The listing builds one solid part. Answer for the finished solid, in the listing's coordinates (mm). Face numbers are marked on the shaded views. A direction names the side the tool comes from. Round coordinates to 2 decimals unless told otherwise and drop trailing zeros. Order: outer loops, then holes, each group sorted by start corner. A loop starts at its lowest first (then second) coordinate and runs counter-clockwise, first axis right, second up. Notation, with made-up numbers: (12.25, 29.25) -> (23.25, 29.25) arc R23 cw to (23.25, 39.25) -> close; hole circle Ø1 at (81, 71.5). An arc over 180 degrees is marked (long way). Answer in a Markdown table with one row per item. Add a question column.
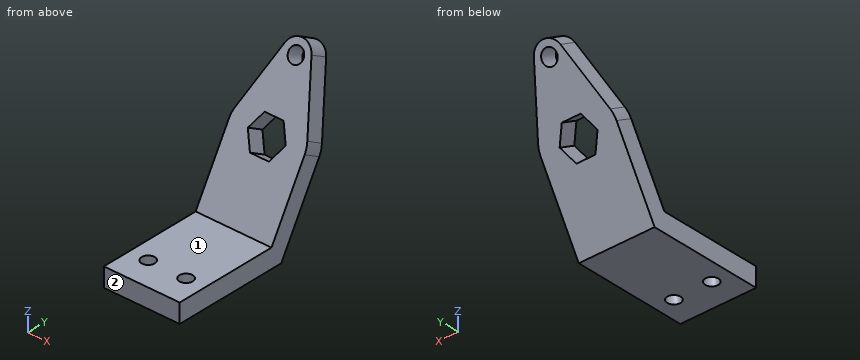
```python
from build123d import *

# Parameters (mm, degrees)
EXTRUDE_THIN1_DEPTH = 20
CUT_EXTRUDE1_REACH  = 104.251
SKETCH2_R           = 3.5
CUT_EXTRUDE9_DEPTH  = 10
SKETCH6_R           = 4
CUT_EXTRUDE10_DEPTH = 10


with BuildPart() as part:
    # Sketch1 → Extrude-Thin1 (new, symmetric)
    with BuildSketch(Plane(origin=(0, 0, 0), x_dir=(0, 0, -1), z_dir=(1, 0, 0))):
        Polygon((0, -60), (0, 0), (-75.344210129, 43.5), (-80.344210129, 34.839745962), (-10, -5.773502692), (-10, -60), align=None)
    extrude(amount=EXTRUDE_THIN1_DEPTH, both=True)

    # Sketch2 → Cut-Extrude1 (cut, up to next)
    with BuildSketch(Plane(origin=(0, 0, 0), x_dir=(-1, 0, 0), z_dir=(0, 0, -1)), mode=Mode.PRIVATE) as cut_extrude1_sk1:
        with Locations((-10, -45)):
            Circle(SKETCH2_R)
    cut_extrude1_tool1 = extrude(cut_extrude1_sk1.sketch, amount=-CUT_EXTRUDE1_REACH, mode=Mode.PRIVATE) & part.part
    # Sketch2 → Cut-Extrude1 (cut, up to next)
    with BuildSketch(Plane(origin=(0, 0, 0), x_dir=(-1, 0, 0), z_dir=(0, 0, -1)), mode=Mode.PRIVATE) as cut_extrude1_sk2:
        with Locations(Location((10, -45, 0), (0, 0, 180))):
            Circle(SKETCH2_R)
    cut_extrude1_tool2 = extrude(cut_extrude1_sk2.sketch, amount=-CUT_EXTRUDE1_REACH, mode=Mode.PRIVATE) & part.part
    add(cut_extrude1_tool1.solids().sort_by_distance((10, -45, 0))[0], mode=Mode.SUBTRACT)
    add(cut_extrude1_tool2.solids().sort_by_distance((-10, -45, 0))[0], mode=Mode.SUBTRACT)

    # Sketch3 → Cut-Extrude9 (cut)
    with BuildSketch(Plane(origin=(0, 0, 0), x_dir=(1, 0, 0), z_dir=(0, 0.8660254037844398, -0.499999999999998))):
        Polygon((29.732274902, -45), (20, -45), (20, -87), (9.8e-08, -87), (-20, -87), (-20, -45), (-32.034408351, -45), (-32.034408351, -100.781822996), (29.732274902, -100.781822996), align=None)
        with BuildLine():
            ThreePointArc((-19.034409454, -50.29484195), (-19.756628033, -47.691083257), (-20, -45))
            Line((-20, -45), (-20, -87))
            Line((-20, -87), (9.8e-08, -87))
            ThreePointArc((9.8e-08, -87), (-4.265814225, -85.668697512), (-7.017204727, -82.147420975))
            Line((-7.017204727, -82.147420975), (-19.034409454, -50.29484195))
        make_face()
        with BuildLine():
            Line((20, -87), (20, -45))
            ThreePointArc((20, -45), (19.756628033, -47.691083257), (19.034409454, -50.29484195))
            Line((19.034409454, -50.29484195), (7.017204727, -82.147420975))
            ThreePointArc((7.017204727, -82.147420975), (4.265814305, -85.668697457), (9.8e-08, -87))
            Line((9.8e-08, -87), (20, -87))
        make_face()
    extrude(amount=-CUT_EXTRUDE9_DEPTH, mode=Mode.SUBTRACT)

    # Sketch6 → Cut-Extrude10 (cut)
    with BuildSketch(Plane(origin=(0, 0, 0), x_dir=(1, 0, 0), z_dir=(0, 0.8660254037844398, -0.499999999999998))):
        with Locations(Location((0, -79.5, 0), (0, 0, 270))):
            Circle(SKETCH6_R)
        Polygon((10, -45), (5, -36.339745962), (-5, -36.339745962), (-10, -45), (-5, -53.660254038), (5, -53.660254038), align=None)
    extrude(amount=-CUT_EXTRUDE10_DEPTH, mode=Mode.SUBTRACT)


solid = part.part
```
Item 1: The part is cut by section B-B, the plane x = 11.5. Give the vertices of the cut face in (y, z).
Item 2: The part is cut by section A-A, the plane y = -45. Give the vertices of the cut face in (x, z), and give its area (3 significant figures).
Item 3: The part is cut by section D-D, the plane z = 6.5. Give the vertices of the cut face in (x, y), and give its area (3 significant figures).
Item 4: The part is cut by section C-C, the plane z = 50. Give the vertices of the cut face in (x, y).
Item 5: Find the intervals of material crossed by probe 1 along Z at (x, y) = (8, -13); probe 2 along X at (y, z) = (22, 39); probe 3 along X at (y, z) = (31, 72.5), in increasing order. Write a range as [from, to].
Item 6: Flat-ended cylindrical pins translate along their axes: P1, Ø5, axis at x = -10.5, y = 21.5, coming from the -Z side; P2, Ø8, axis at x = -11.5, y = -19.5, coming from the +Z side; P3, Ø8, axis at x = 2.5, y = 22, coming from the -Z side. Find the tip coordinate at first contact, or state that the pin passes through.
Item 7: A tool of negligible diameter and unlimited length cuts with its end or side. For the marked faces 1 and 2, from which of +Z, -Z, +X, -X, +Y, -Y can it reach the whole face along a straight path? Write none if from no direction.
Resolved:
| question | item | result |
|---|---|---|
| 1 | outline | (-60, 0) -> (-48.16, 0) -> (-48.16, 10) -> (-60, 10) -> close; (-41.84, 0) -> (0, 0) -> (35.13, 60.85) -> (26.47, 65.85) -> (-5.77, 10) -> (-41.84, 10) -> close |
| 2 | outline | (-20, 0) -> (-13.5, 0) -> (-13.5, 10) -> (-20, 10) -> close; (-6.5, 0) -> (6.5, 0) -> (6.5, 10) -> (-6.5, 10) -> close; (13.5, 0) -> (20, 0) -> (20, 10) -> (13.5, 10) -> close |
| 2 | area | 260 mm2 |
| 3 | outline | (-20, -60) -> (20, -60) -> (20, 3.75) -> (-20, 3.75) -> close; hole circle Ø7 at (-10, -45); hole circle Ø7 at (10, -45) |
| 3 | area | 2,470 mm2 |
| 4 | outline | (-18.41, 17.32) -> (-5.98, 17.32) -> (-5, 20.72) -> (5, 20.72) -> (5.98, 17.32) -> (18.41, 17.32) -> (16.23, 28.87) -> (-16.23, 28.87) -> close |
| 5 | probe 1 | [0, 10] |
| 5 | probe 2 | [-20, -9.87], [9.87, 20] |
| 5 | probe 3 | [-8.47, -3.81], [3.81, 8.47] |
| 6 | P1 | z = 32.91 |
| 6 | P2 | z = 10 |
| 6 | P3 | z = 31.18 |
| 7 | face 1 | +Z, +X, -X, -Y |
| 7 | face 2 | +Z, -Z, +X, -X, -Y |
